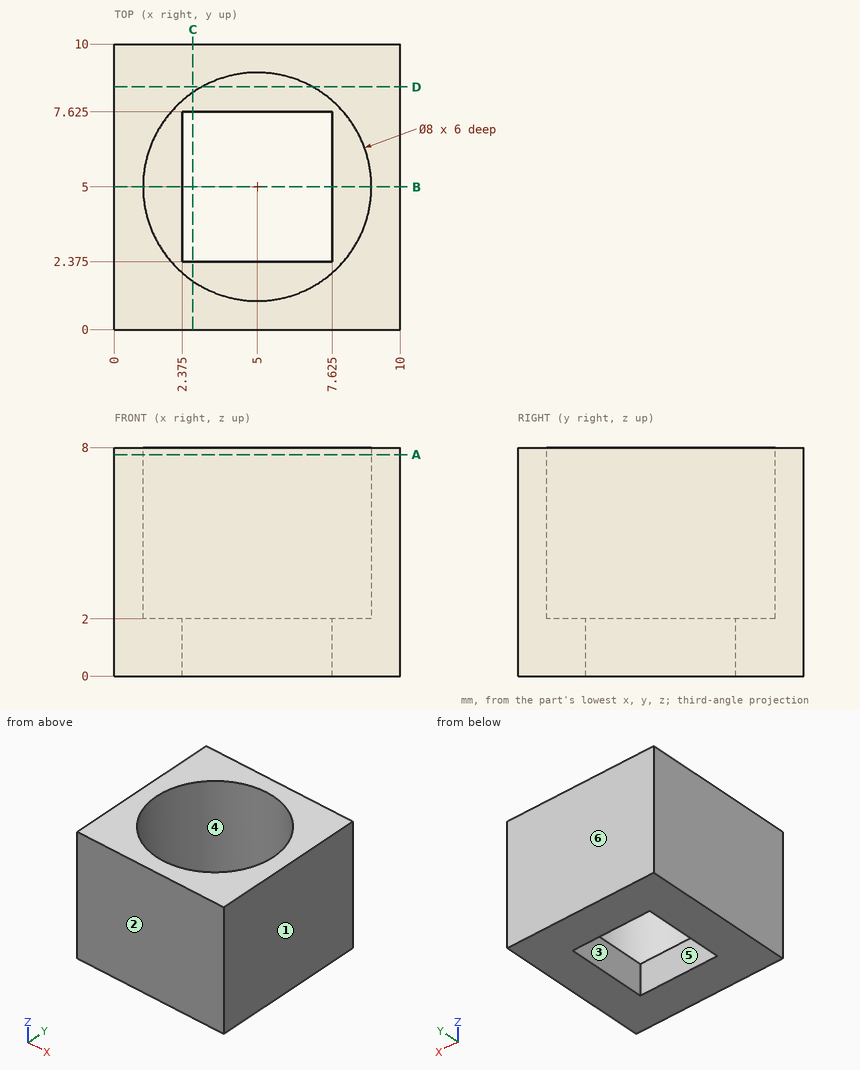
For this review, use the dimensioned drawing (mm, ordinates from the lowest corner) and the shaded views. A direction names the side the tool comes from. Round coordinates to 2 decimals unless told otherwise and drop trailing zeros. Write each loop counter-clockwise with the first axis right and the second up, starting at its lowest first coordinate (ties: lowest second). Pieces come first, ordered by that corner, then holes. Notation, with made-up numbers: (-10, -29.5) -> (37, -29.5) arc R8 ccw to (37, -16.5) -> close; hole circle Ø9 at (-10, 2.5). An arc over 180 degrees is marked (long way). Use CSV: the item, a comma, the result in double quotes.
(1) For the marked faces 4, 5 and 6, list the 3-axis set-ups (+Z, -Z, +X, -X, +Y, -Y) from which the entire face can be reached by the end or side of a thin tool; tool diameter is ignored.
Computed values:
face 4,"+Z"
face 5,"+Z, -Z"
face 6,"+Z, -Z, +X, -X, +Y"
(2) Consider section D-D, the plane y = 8.5. Give the boundary of the cut face in (x, z), plus the area to 3 significant figures.
Computed values:
outline,"(0, 0) -> (10, 0) -> (10, 8) -> (6.94, 8) -> (6.94, 2) -> (3.06, 2) -> (3.06, 8) -> (0, 8) -> close"
area,"56.8 mm²"
(3) Consider section B-B, the plane y = 5. Give the boundary of the cut face in (x, z) (3 decimals), plus the area to 3 significant figures.
Computed values:
outline,"(0, 0) -> (2.375, 0) -> (2.375, 2) -> (1, 2) -> (1, 8) -> (0, 8) -> close; (7.625, 0) -> (10, 0) -> (10, 8) -> (9, 8) -> (9, 2) -> (7.625, 2) -> close"
area,"21.5 mm²"
(4) Consider section C-C, the plane x = 2.75. Give the boundary of the cut face in (y, z) (3 decimals), plus the area to 3 significant figures.
Computed values:
outline,"(0, 0) -> (2.375, 0) -> (2.375, 2) -> (1.693, 2) -> (1.693, 8) -> (0, 8) -> close; (7.625, 0) -> (10, 0) -> (10, 8) -> (8.307, 8) -> (8.307, 2) -> (7.625, 2) -> close"
area,"29.8 mm²"
(5) To check wall thickness, follow L1, parallel to Y at x = 5, z = 3.6; L2, parallel to Z at x = 5.75, y = 2.25; L3, parallel to X at y = 6.25, z = 5.5. State the ranges of each line that lie inside material, in increasing order. Write a range as [from, to].
Computed values:
L1,"[0, 1], [9, 10]"
L2,"[0, 2]"
L3,"[0, 1.2], [8.8, 10]"
(6) Consider section A-A, the plane z = 7.75. Give the boundary of the cut face in (x, y), plus the area to 3 significant figures.
Computed values:
outline,"(0, 0) -> (10, 0) -> (10, 10) -> (0, 10) -> close; hole circle Ø8 at (5, 5)"
area,"49.7 mm²"
(7) Draft analysis for pull direction Y (two halves, no side actions). For the marked faces 1, 2 and 3, state which applies: +Y half, -Y half, draft (parallel to the pull), parting line (faces both ways), or undercut.
Computed values:
face 1,"draft"
face 2,"-Y half"
face 3,"undercut"
